The figure shows three views and two pictorial views of one solid part (mm, origin at its lowest corner). Answer the questions. A direction names the side the tool comes from. Coordinates: 2 decimals unless noted, no trailing zeros. Loops run counter-clockwise (first coordinate to the right, second up) from the corner with the lowest first, then second, coordinate; pieces in that order, holes last.
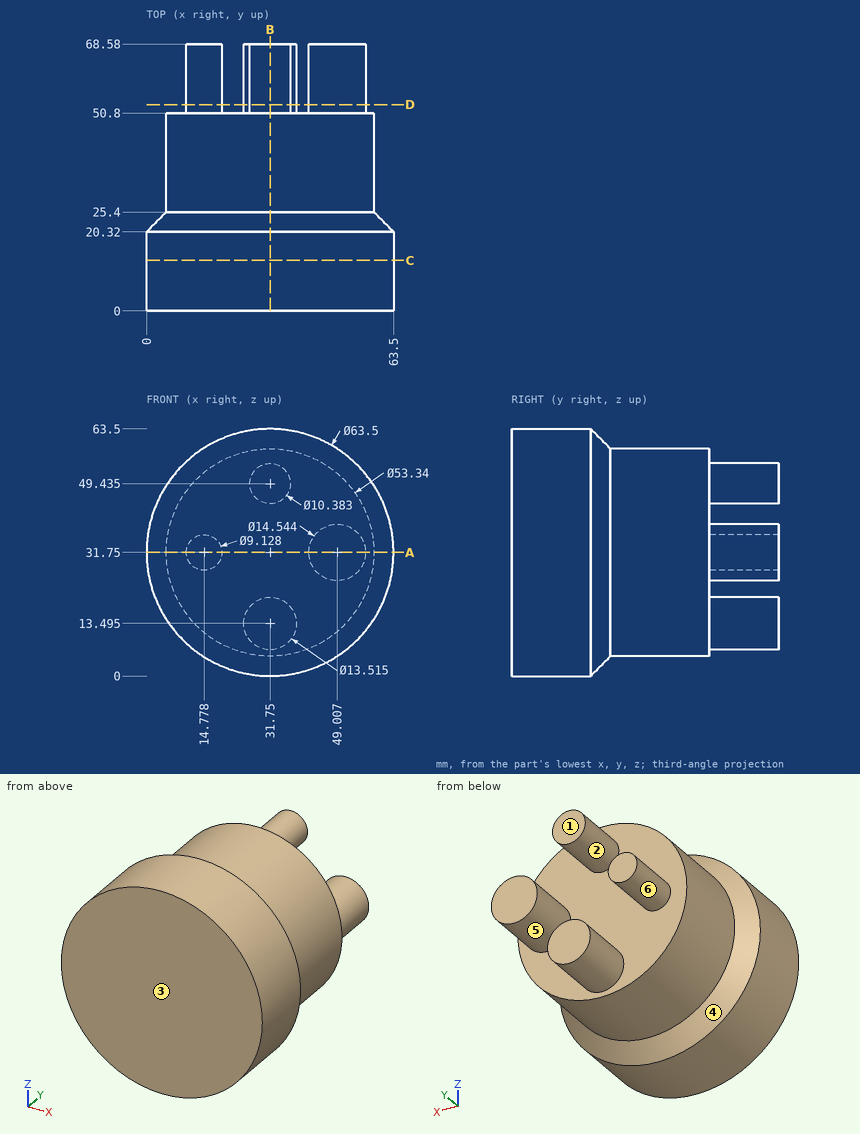
1. A cutting plane is placed at D-D, the plane y = 53. Count the separate pieces of the cut face and the enclosed holes in it, then the cut area to 3 significant figures.
2. A cutting plane is placed at C-C, the plane y = 13. Give the vertices of the cut face in (x, z), then the cut area to 3 significant figures.
3. Each of these flat-tipped pins is pushed along its axis until it touches: P1, Ø3, axis at x = 51.5, y = 61, coming from the -Z side; P2, Ø12, axis at y = 37, z = 31.5, coming from the +X side; P3, Ø1, axis at x = 49, y = 11, coming from the -Z side; P4, Ø3, axis at x = 47.5, z = 24, coming from the +Y side. Where does it stop, or does it pass through?
4. Straight lines are drawn through the part: probe 1 along X at (y, z) = (53, 31.5) (1 decimal); probe 2 along Y at (x, z) = (38, 18); probe 3 along Z at (x, y) = (35.5, 57.5) (1 decimal). For each, find the intervals that lie inside material, in ascending order.
5. For the marked faces 1 and 2, determine the directions among +Z, -Z, +X, -X, +Y, -Y from which every point of the face is accessible in a straight line to the end or side of a thin tool.
6. A cutting plane is placed at A-A, the plane z = 31.75. Give the vertices of the cut face in (x, y) (1 decimal).
7. Determine the mould class of the marked faces 3, 4, 5 and 6 for opening direction X: released by +X, released by -X, zero draft, split by the parting line, or undercut.
8. A cutting plane is placed at B-B, the plane x = 31.75. Give the vertices of the cut face in (y, z), then the cut area to 3 significant figures.
Answers below:
1. separate pieces: 4
1. enclosed holes: 0
1. area: 460 mm2
2. outline: circle Ø63.5 at (31.75, 31.75)
2. area: 3,170 mm2
3. P1: stops at z = 24.55
3. P2: stops at x = 58.42
3. P3: stops at z = 4.78
3. P4: stops at y = 68.58
4. probe 1: x = 10.2 to 19.3, 41.7 to 56.3
4. probe 2: y = 0 to 50.8
4. probe 3: z = 7.9 to 19.1, 45.8 to 53
5. face 1: +Z, -Z, +X, -X, +Y
5. face 2: +Y
6. outline: (0, 0) - (63.5, 0) - (63.5, 20.3) - (58.4, 25.4) - (58.4, 50.8) - (56.3, 50.8) - (56.3, 68.6) - (41.7, 68.6) - (41.7, 50.8) - (19.3, 50.8) - (19.3, 68.6) - (10.2, 68.6) - (10.2, 50.8) - (5.1, 50.8) - (5.1, 25.4) - (0, 20.3) - close
7. face 3: zero draft
7. face 4: split by the parting line
7. face 5: undercut
7. face 6: undercut
8. outline: (0, 0) - (20.32, 0) - (25.4, 5.08) - (50.8, 5.08) - (50.8, 6.74) - (68.58, 6.74) - (68.58, 20.25) - (50.8, 20.25) - (50.8, 44.24) - (68.58, 44.24) - (68.58, 54.63) - (50.8, 54.63) - (50.8, 58.42) - (25.4, 58.42) - (20.32, 63.5) - (0, 63.5) - close
8. area: 3,370 mm2
